from build123d import *

# Parameters (mm, degrees)
SKETCH_W     = 43
SKETCH_H     = 43
PAD_DEPTH    = 20
SKETCH001_R  = 11
POCKET_DEPTH = 5
POCKET_TAPER = 30
FILLET_R     = 3


with BuildPart() as part:
    # Sketch → Pad (new body)
    with BuildSketch(Plane.XY):
        Rectangle(SKETCH_W, SKETCH_H)
    extrude(amount=PAD_DEPTH)

    # Sketch001 (on Face6 of Pad) → Pocket (cut)
    with BuildSketch(Plane.XY.offset(20)):
        Circle(SKETCH001_R)
    extrude(amount=-POCKET_DEPTH, taper=POCKET_TAPER, mode=Mode.SUBTRACT)

    # Fillet
    fillet_edges = [part.edges().sort_by_distance(p)[0] for p in [
        (21.5, -21.5, 10),
        (21.5, 21.5, 10),
        (-21.5, -21.5, 10),
        (-21.5, 21.5, 10),
    ]]
    fillet(fillet_edges, radius=FILLET_R)


solid = part.part
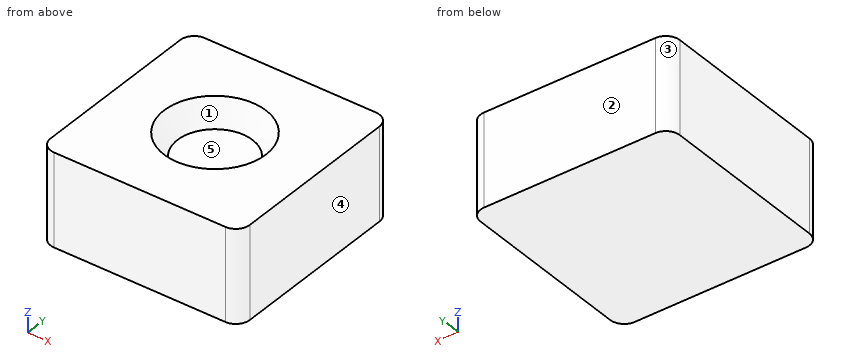
For this review, take the finished solid that the model builds, in its own axes (mm). Face numbers are marked on the shaded views. A direction names the side the tool comes from. Give positions to 0.01 mm unless a question says otherwise; leave off trailing zeros. Loops run counter-clockwise (first coordinate to the right, second up) from the corner with the lowest first, then second, coordinate; pieces in that order, holes last.
Item 1: Take a section at B-B, the plane x = 0. State the section outline as (y, z) points, and give its area (3 significant figures).
Item 2: Draft analysis for pull direction X (two halves, no side actions). For the marked faces 1, 2 and 3, state which applies: +X half, -X half, draft (parallel to the pull), parting line (faces both ways), or undercut.
Item 3: Tool access review of the marked faces 4 and 5: name each direction out of +Z, -Z, +X, -X, +Y, -Y from which nothing blocks a thin tool from reaching the whole face with its end or side.
Item 4: For line 1 along Y through (x, z) = (-2.5, 18); line 2 along X through (y, z) = (1.5, 17.75); line 3 along Y through (x, z) = (3, 17.25), list the stretches that pass through material, from the lowest coordinate up.
Item 5: Take a section at A-A, the plane z = 17.5. State the section outline as (x, y) points.
Calculated:
1. outline: (-21.5, 0) - (21.5, 0) - (21.5, 20) - (11, 20) - (8.11, 15) - (-8.11, 15) - (-11, 20) - (-21.5, 20) - close
1. area: 764 mm2
2. face 1: undercut
2. face 2: draft
2. face 3: -X half
3. face 4: +Z, -Z, +X, +Y, -Y
3. face 5: +Z
4. line 1: y = -21.5 to -9.52, 9.52 to 21.5
4. line 2: x = -21.5 to -9.58, 9.58 to 21.5
4. line 3: y = -21.5 to -8.92, 8.92 to 21.5
5. outline: (-21.5, -18.5) arc R3 ccw to (-18.5, -21.5) - (18.5, -21.5) arc R3 ccw to (21.5, -18.5) - (21.5, 18.5) arc R3 ccw to (18.5, 21.5) - (-18.5, 21.5) arc R3 ccw to (-21.5, 18.5) - close; hole circle Ø19.11 at (0, 0)
